Input: part model. Units: mm. Frame: model coordinates. A direction names the side the tool comes from. Coordinates: 2 decimals unless noted, no trailing zeros. Loops run counter-clockwise (first coordinate to the right, second up) from the corner with the lowest first, then second, coordinate; pieces in that order, holes last. Notation, with made-up numbers: (19.5, 12) -> (51.5, 12) arc R26 ccw to (51.5, 26) -> close; hole circle Ø1 at (88.25, 83.25). An arc over 180 degrees is marked (long way). Put each result on its own line as item: value. Start each with the question number.
1) Cut plane B-B (x = 250). Return the cut outline in (y, z), plus the area to 3 significant figures.
2) Cut plane A-A (z = -206.5). Return the cut outline in (x, y), plus the area to 3 significant figures.
3) Cut plane C-C (y = 350). State how many separate pieces and enclosed holes the cut face has, plus the area to 3 significant figures.
4) Pull-direction query (X, two-part tool) for faces 4 (the flat face through (-287.488, 311, 18)), 5 (the flat face through (926, 678, 0)), 6 (the flat face through (926, 1104.341, 86)), 7 (the flat face through (2150.912, 311, 18)); classes: pulls with the +X half, pulls with the -X half, needs draft (parallel to the pull), parting line crosses it, or undercut.
5) Set-up query: faces 1 (the flat face through (926, 1078.941, 236)), 2 (the flat face through (926, 1085, 279.4)), 3 (the flat face through (926, 678, 25.4)). Return all of +Z, -Z, +X, -X, +Y, -Y with unobstructed straight access to the full face (end or side cutting, diameter ignored); none if empty.
6) Material intervals for L1, parallel to Y at x = 107.5, z = 2; L2, parallel to Z at x = 169.5, y = 686, sorted ascending.
7) Contact query for a flat-ended pin moving along its axis: P1, Ø5, axis at x = 818.5, z = 28.5, coming from the +Y side (3 decimals). Output: stop coordinate, or through.
from build123d import *

# Parameters (mm, degrees)
F0_W     = 25.4
F0_H     = 25.4
F0_W_2   = 376.7666666667
F0_H_2   = 372.5333333333
F1_DEPTH = 25.4
F2_DEPTH = 330.2
F3_DEPTH = 254
F4_W     = 2438.4
F4_H     = 1219.2
F4_W_2   = 2387.6
F4_H_2   = 1168.4
F5_DEPTH = 25.4


with BuildPart() as f1:
    # F0 (on Top) → F1 (new body)
    with BuildSketch(Plane.XY):
        with Locations((931.7122847671, -102.1590246889)):
            Rectangle(F0_W, F0_H)
        Polygon((919.0122847671, 1104.3409753111), (-262.0877152329, 1104.3409753111), (-262.0877152329, 1078.9409753111), (-287.4877152329, 1078.9409753111), (-287.4877152329, -89.4590246889), (-262.0877152329, -89.4590246889), (-262.0877152329, -114.8590246889), (919.0122847671, -114.8590246889), (919.0122847671, -89.4590246889), (944.4122847671, -89.4590246889), (944.4122847671, -114.8590246889), (2125.5122847671, -114.8590246889), (2125.5122847671, -89.4590246889), (2150.9122847671, -89.4590246889), (2150.9122847671, 1078.9409753111), (2125.5122847671, 1078.9409753111), (2125.5122847671, 1104.3409753111), (944.4122847671, 1104.3409753111), (944.4122847671, 1078.9409753111), (919.0122847671, 1078.9409753111), align=None)
        with Locations((-73.7043818996, 96.8076419778)):
            Rectangle(F0_W_2, F0_H_2, mode=Mode.SUBTRACT)
        with Locations((328.4622847671, 96.8076419778)):
            Rectangle(F0_W_2, F0_H_2, mode=Mode.SUBTRACT)
        with Locations((730.6289514337, 96.8076419778)):
            Rectangle(F0_W_2, F0_H_2, mode=Mode.SUBTRACT)
        with Locations((-73.7043818996, 494.7409753111)):
            Rectangle(F0_W_2, F0_H_2, mode=Mode.SUBTRACT)
        with Locations((1132.7956181004, 96.8076419778)):
            Rectangle(F0_W_2, F0_H_2, mode=Mode.SUBTRACT)
        with Locations((1534.9622847671, 96.8076419778)):
            Rectangle(F0_W_2, F0_H_2, mode=Mode.SUBTRACT)
        with Locations((1937.1289514337, 96.8076419778)):
            Rectangle(F0_W_2, F0_H_2, mode=Mode.SUBTRACT)
        with Locations((1534.9622847671, 494.7409753111)):
            Rectangle(F0_W_2, F0_H_2, mode=Mode.SUBTRACT)
        with Locations((1937.1289514337, 494.7409753111)):
            Rectangle(F0_W_2, F0_H_2, mode=Mode.SUBTRACT)
        with Locations((328.4622847671, 494.7409753111)):
            Rectangle(F0_W_2, F0_H_2, mode=Mode.SUBTRACT)
        with Locations((730.6289514337, 494.7409753111)):
            Rectangle(F0_W_2, F0_H_2, mode=Mode.SUBTRACT)
        with Locations((-73.7043818996, 892.6743086444)):
            Rectangle(F0_W_2, F0_H_2, mode=Mode.SUBTRACT)
        with Locations((328.4622847671, 892.6743086444)):
            Rectangle(F0_W_2, F0_H_2, mode=Mode.SUBTRACT)
        with Locations((730.6289514337, 892.6743086444)):
            Rectangle(F0_W_2, F0_H_2, mode=Mode.SUBTRACT)
        with Locations((1132.7956181004, 494.7409753111)):
            Rectangle(F0_W_2, F0_H_2, mode=Mode.SUBTRACT)
        with Locations((1132.7956181004, 892.6743086444)):
            Rectangle(F0_W_2, F0_H_2, mode=Mode.SUBTRACT)
        with Locations((1534.9622847671, 892.6743086444)):
            Rectangle(F0_W_2, F0_H_2, mode=Mode.SUBTRACT)
        with Locations((1937.1289514337, 892.6743086444)):
            Rectangle(F0_W_2, F0_H_2, mode=Mode.SUBTRACT)
        with Locations((-274.7877152329, -102.1590246889)):
            Rectangle(F0_W, F0_H)
        with Locations((931.7122847671, 1091.6409753111)):
            Rectangle(F0_W, F0_H)
        with Locations((-274.7877152329, 1091.6409753111)):
            Rectangle(F0_W, F0_H)
        with Locations((2138.2122847671, -102.1590246889)):
            Rectangle(F0_W, F0_H)
        with Locations((2138.2122847671, 1091.6409753111)):
            Rectangle(F0_W, F0_H)
    extrude(amount=F1_DEPTH)

    # F0 (on Top) → F2 (join)
    with BuildSketch(Plane.XY):
        with Locations((-274.7877152329, 1091.6409753111)):
            Rectangle(F0_W, F0_H)
        with Locations((-274.7877152329, -102.1590246889)):
            Rectangle(F0_W, F0_H)
        with Locations((931.7122847671, -102.1590246889)):
            Rectangle(F0_W, F0_H)
        with Locations((2138.2122847671, -102.1590246889)):
            Rectangle(F0_W, F0_H)
        with Locations((2138.2122847671, 1091.6409753111)):
            Rectangle(F0_W, F0_H)
        with Locations((931.7122847671, 1091.6409753111)):
            Rectangle(F0_W, F0_H)
    extrude(amount=-F2_DEPTH)

    # F0 (on Top) → F3 (join)
    with BuildSketch(Plane.XY):
        with Locations((-274.7877152329, 1091.6409753111)):
            Rectangle(F0_W, F0_H)
        with Locations((931.7122847671, 1091.6409753111)):
            Rectangle(F0_W, F0_H)
        with Locations((-274.7877152329, -102.1590246889)):
            Rectangle(F0_W, F0_H)
        with Locations((931.7122847671, -102.1590246889)):
            Rectangle(F0_W, F0_H)
        with Locations((2138.2122847671, -102.1590246889)):
            Rectangle(F0_W, F0_H)
        with Locations((2138.2122847671, 1091.6409753111)):
            Rectangle(F0_W, F0_H)
    extrude(amount=F3_DEPTH)

    # F4 (on face) → F5 (join)
    with BuildSketch(Plane.XY.offset(254)):
        with Locations((931.7122847671, 494.7409753111)):
            Rectangle(F4_W, F4_H)
        with Locations((931.7122847671, 494.7409753111)):
            Rectangle(F4_W_2, F4_H_2, mode=Mode.SUBTRACT)
    extrude(amount=F5_DEPTH)


solid = f1.part
Results found:
1. outline: (-114.86, 0) -> (-89.46, 0) -> (-89.46, 25.4) -> (-114.86, 25.4) -> close; (-114.86, 254) -> (-89.46, 254) -> (-89.46, 279.4) -> (-114.86, 279.4) -> close; (283.07, 0) -> (308.47, 0) -> (308.47, 25.4) -> (283.07, 25.4) -> close; (681.01, 0) -> (706.41, 0) -> (706.41, 25.4) -> (681.01, 25.4) -> close; (1078.94, 0) -> (1104.34, 0) -> (1104.34, 25.4) -> (1078.94, 25.4) -> close; (1078.94, 254) -> (1104.34, 254) -> (1104.34, 279.4) -> (1078.94, 279.4) -> close
1. area: 3,870 mm2
2. outline: (-287.49, -114.86) -> (-262.09, -114.86) -> (-262.09, -89.46) -> (-287.49, -89.46) -> close; (-287.49, 1078.94) -> (-262.09, 1078.94) -> (-262.09, 1104.34) -> (-287.49, 1104.34) -> close; (919.01, -114.86) -> (944.41, -114.86) -> (944.41, -89.46) -> (919.01, -89.46) -> close; (919.01, 1078.94) -> (944.41, 1078.94) -> (944.41, 1104.34) -> (919.01, 1104.34) -> close; (2125.51, -114.86) -> (2150.91, -114.86) -> (2150.91, -89.46) -> (2125.51, -89.46) -> close; (2125.51, 1078.94) -> (2150.91, 1078.94) -> (2150.91, 1104.34) -> (2125.51, 1104.34) -> close
2. area: 3,870 mm2
3. separate pieces: 9
3. enclosed holes: 0
3. area: 5,810 mm2
4. face 4: pulls with the -X half
4. face 5: undercut
4. face 6: needs draft
4. face 7: pulls with the +X half
5. face 1: +Z
5. face 2: +Z, +X, -X, +Y, -Y
5. face 3: none
6. L1: y = -114.86 to -89.46, 283.07 to 308.47, 681.01 to 706.41, 1078.94 to 1104.34
6. L2: z = 0 to 25.4
7. P1: passes through
